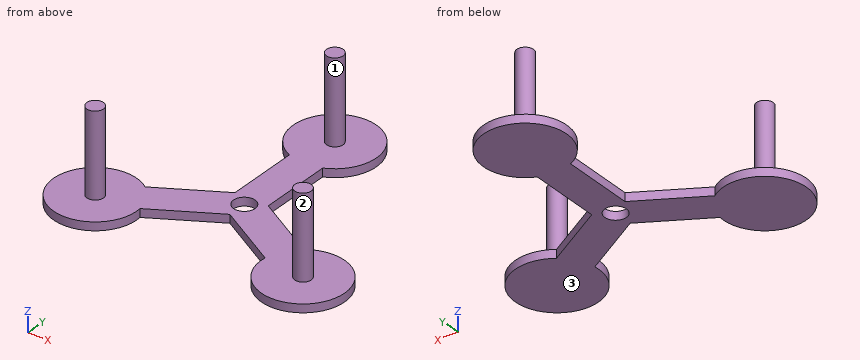
from build123d import *

# Parameters (mm, degrees)
BOSS_EXTRUDE2_DEPTH = 10
SKETCH3_R           = 50
BOSS_EXTRUDE3_DEPTH = 10
SKETCH4_R           = 10
BOSS_EXTRUDE4_DEPTH = 90
CUT_EXTRUDE1_START  = -30
SKETCH5_R           = 10
CUT_EXTRUDE1_DEPTH  = 30
SKETCH6_R           = 13
CUT_EXTRUDE2_DEPTH  = 10
SKETCH7_R           = 10
BOSS_EXTRUDE5_DEPTH = 30
SKETCH9_R           = 10
BOSS_EXTRUDE6_DEPTH = 10
SKETCH10_R          = 10
BOSS_EXTRUDE7_DEPTH = 10
SKETCH11_R          = 10
BOSS_EXTRUDE8_DEPTH = 10


with BuildPart() as part:
    # Sketch1 → Boss-Extrude2 (new body)
    with BuildSketch(Plane.XY):
        Polygon((20, 144), (-20, 144), (-20, 11.547005384), (-134.707658145, -54.679491924), (-114.707658145, -89.320508076), (0, -23.094010768), (114.707658145, -89.320508076), (134.707658145, -54.679491924), (20, 11.547005384), align=None)
    extrude(amount=BOSS_EXTRUDE2_DEPTH)

    # Sketch3 → Boss-Extrude3 (add)
    with BuildSketch(Plane.XY.offset(10)):
        with Locations((-124.707658145, -72)):
            Circle(SKETCH3_R)
        with Locations((0, 144)):
            Circle(SKETCH3_R)
        with Locations((124.707658145, -72)):
            Circle(SKETCH3_R)
    extrude(amount=-BOSS_EXTRUDE3_DEPTH)

    # Sketch4 → Boss-Extrude4 (add)
    with BuildSketch(Plane.XY.offset(10)):
        with Locations(Location((0, 144, 0), (0, 0, 180))):
            Circle(SKETCH4_R)
        with Locations(Location((124.707658145, -72, 0), (0, 0, 180))):
            Circle(SKETCH4_R)
        with Locations(Location((-124.707658145, -72, 0), (0, 0, 180))):
            Circle(SKETCH4_R)
    extrude(amount=BOSS_EXTRUDE4_DEPTH)

    # Sketch5 → Cut-Extrude1 (cut)
    with BuildSketch(Plane.XY.offset(100).offset(CUT_EXTRUDE1_START)):
        with Locations(Location((0, 144, 0), (0, 0, 180))):
            Circle(SKETCH5_R)
    extrude(amount=CUT_EXTRUDE1_DEPTH, mode=Mode.SUBTRACT)

    # Sketch6 → Cut-Extrude2 (cut)
    with BuildSketch(Plane.XY.offset(10)):
        Circle(SKETCH6_R)
    extrude(amount=-CUT_EXTRUDE2_DEPTH, mode=Mode.SUBTRACT)

    # Sketch7 → Boss-Extrude5 (add)
    with BuildSketch(Plane.XY.offset(70)):
        with Locations(Location((0, 144, 0), (0, 0, 180))):
            Circle(SKETCH7_R)
    extrude(amount=BOSS_EXTRUDE5_DEPTH)

    # Sketch9 → Boss-Extrude6 (add)
    with BuildSketch(Plane.XY.offset(100)):
        with Locations(Location((0, 144, 0), (0, 0, 180))):
            Circle(SKETCH9_R)
    extrude(amount=BOSS_EXTRUDE6_DEPTH)

    # Sketch10 → Boss-Extrude7 (add)
    with BuildSketch(Plane.XY.offset(100)):
        with Locations(Location((-124.707658145, -72, 0), (0, 0, 180))):
            Circle(SKETCH10_R)
    extrude(amount=BOSS_EXTRUDE7_DEPTH)

    # Sketch11 → Boss-Extrude8 (add)
    with BuildSketch(Plane.XY.offset(100)):
        with Locations(Location((124.707658145, -72, 0), (0, 0, 180))):
            Circle(SKETCH11_R)
    extrude(amount=BOSS_EXTRUDE8_DEPTH)


solid = part.part
Model file for the job. Use its own axes, mm. Face numbers are marked on the shaded views. Give positions to 0.01 mm unless a question says otherwise; leave off trailing zeros. Loops run counter-clockwise (first coordinate to the right, second up) from the corner with the lowest first, then second, coordinate; pieces in that order, holes last.
Item 1: Slice it at D-D (y = 144). Write the cut outline in (x, z).
Check values:
outline: (-50, 0) - (50, 0) - (50, 10) - (10, 10) - (10, 110) - (-10, 110) - (-10, 10) - (-50, 10) - close
Item 2: Slice it at B-B (y = -72). Write the cut outline in (x, z).
Check values:
outline: (-174.71, 0) - (-74.71, 0) - (-74.71, 10) - (-114.71, 10) - (-114.71, 110) - (-134.71, 110) - (-134.71, 10) - (-174.71, 10) - close; (74.71, 0) - (174.71, 0) - (174.71, 10) - (134.71, 10) - (134.71, 110) - (114.71, 110) - (114.71, 10) - (74.71, 10) - close
Item 3: Drill centre lines: line 1 along Y through (x, z) = (0, 4); line 2 along Z through (x, y) = (-113, -28); line 3 along X through (y, z) = (-63, 15.5). Where is each one in solid material? Low to high.
Check values:
line 1: y = -23.09 to -13, 13 to 194
line 2: z = 0 to 10
line 3: x = -129.07 to -120.35, 120.35 to 129.07
Item 4: Drop flat-ended pins along their axis: P1, Ø5, axis at y = 42, z = 4.5, coming from the +X side; P2, Ø11, axis at y = 60.5, z = 5, coming from the -X side; P3, Ø6, axis at x = 11, z = 93, coming from the -Y side. Give the stop position or say it passes through.
Check values:
P1: stops at x = 20
P2: stops at x = -20
P3: stops at y = 138
Item 5: Slice it at C-C (z = 39). Write the cut outline in (x, y).
Check values:
outline: circle Ø20 at (-124.71, -72); circle Ø20 at (0, 144); circle Ø20 at (124.71, -72)
Item 6: Mould opens along X. For the marked faces 1, 2 and 3 say: +X half, -X half, draft (parallel to the pull), parting line (faces both ways), or undercut.
Check values:
face 1: parting line
face 2: undercut
face 3: draft
Item 7: Slice it at A-A (y = 0). Write the cut outline in (x, z), plus the area to 3 significant figures.
Check values:
outline: (-40, 0) - (-13, 0) - (-13, 10) - (-40, 10) - close; (13, 0) - (40, 0) - (40, 10) - (13, 10) - close
area: 540 mm2
